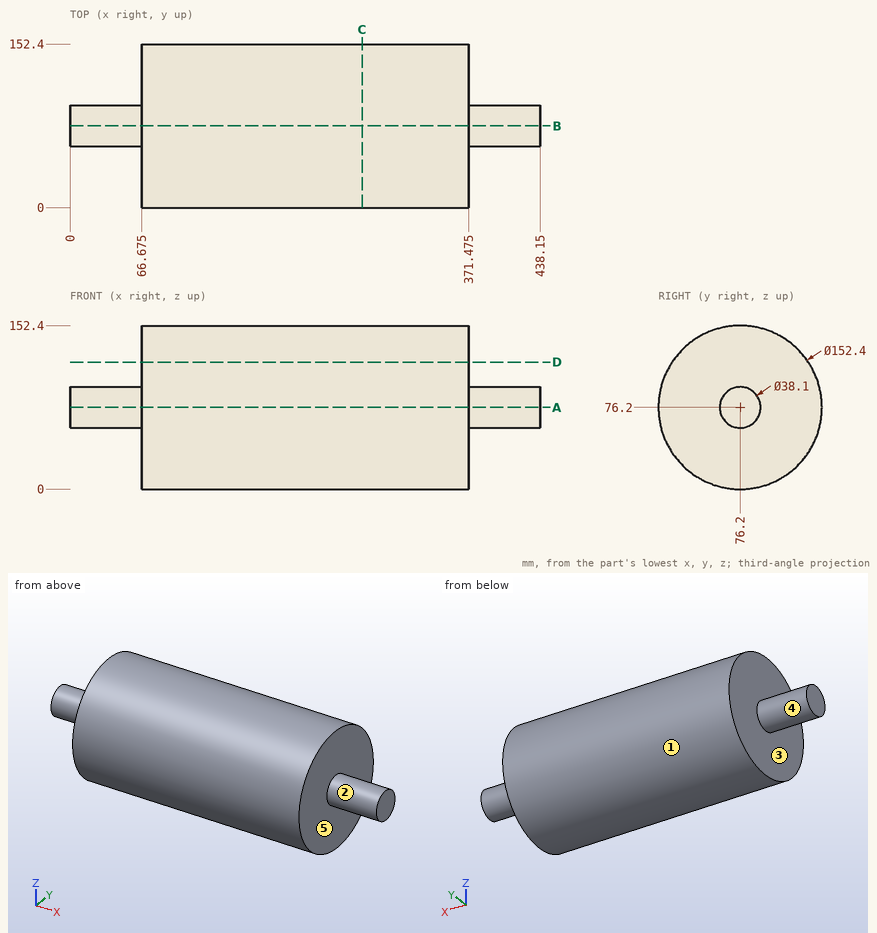
Could you check a few things on this drawing? It's one solid part, dimensions in mm from its lowest x, y, z. A direction names the side the tool comes from. Give positions to 0.01 mm unless a question says otherwise; leave off trailing zeros. Write each loop counter-clockwise with the first axis right and the second up, starting at its lowest first coordinate (ties: lowest second). Pieces come first, ordered by that corner, then holes. Notation, with made-up numbers: M 40.25,14.25 L 78.25,14.25 A17 ccw 78.25,30.25 Z; hole C -24,76.5 d2. An arc over 180 degrees is marked long. Put each result on its own line as item: value. Start each with the question number.
Item 1: If we section it at C-C, the plane x = 272: Write out the boundary of the cut face in (y, z).
Item 2: Will these pins go through, and if not, where does the flat tip stop? pin 1 (12 mm diameter, centred on x = 130.5, z = 65, fed in from -Y); pin 2 (1.5 mm diameter, centred on x = 321, y = 105.5, fed in from -Z); pin 3 (3 mm diameter, centred on y = 73.5, z = 108, fed in from +X) (3 decimals).
Item 3: If we section it at D-D, the plane z = 118.5: Write out the boundary of the cut face in (x, y) (3 decimals), then the cut area to 3 significant figures.
Item 4: I need wall thicknesses on L1, parallel to X at y = 7, z = 72 (3 decimals); L2, parallel to Z at x = 192, y = 76; L3, parallel to Z at x = 279, y = 98.5. Which ranges of each line are inside material? Lowest first, please. Write a range as from..to.
Item 5: If we section it at A-A, the plane z = 76.2: Write out the boundary of the cut face in (x, y) (3 decimals).
Item 6: Thinking about a two-plate mould opening in Z: for the marked faces 4 and 5, which applies, +Z half, -Z half, draft (parallel to the pull), parting line (faces both ways), or undercut?
Item 7: On a 3-axis mill with a long thin cutter (end or side, diameter ignored), from which of +Z, -Z, +X, -X, +Y, -Y can I reach the whole of each face in a straight line? I mean the marked faces 1, 2 and 3. Say none if no direction works.
Values:
1. outline: C 76.2,76.2 d152.4
2. pin 1: y = 0.18
2. pin 2: z = 5.55
2. pin 3: x = 371.475
3. outline: M 66.675,12.819 L 371.475,12.819 L 371.475,139.581 L 66.675,139.581 Z
3. area: 38,600 mm²
4. L1: 66.675..371.475
4. L2: 0..152.4
4. L3: 3.34..149.06
5. outline: M 0,57.15 L 66.675,57.15 L 66.675,0 L 371.475,0 L 371.475,57.15 L 438.15,57.15 L 438.15,95.25 L 371.475,95.25 L 371.475,152.4 L 66.675,152.4 L 66.675,95.25 L 0,95.25 Z
6. face 4: parting line
6. face 5: draft
7. face 1: +X, -X
7. face 2: +X
7. face 3: -X
